Work out the finished part from the listing and answer in its coordinate system (mm). A direction names the side the tool comes from. Coordinates: 2 decimals unless noted, no trailing zeros. Order: outer loops, then holes, each group sorted by start corner. A loop starts at its lowest first (then second) coordinate and runs counter-clockwise, first axis right, second up. Notation, with made-up numbers: (3.25, -37.5) -> (32.25, -37.5) arc R16 ccw to (32.25, -19.5) -> close; hole circle Ø10 at (61.25, 43.25). An arc over 180 degrees is marked (long way). Write item = value, one per line. Start each with the question number.
Q1. The part is cut by section C-C, the plane y = -16. Determine the outline of the cut face in (x, z).
Q2. Which of the six approach directions +Z, -Z, +X, -X, +Y, -Y give full straight-line access (tool end or side, diameter ignored) to faces 1 (the flat face through (249, 24.789, 29)), 2 (the flat face through (247.33, 20.74, 34.51)), 3 (the cylindrical face through (243.607, 30.111, 40.975))?
Q3. The part is cut by section A-A, the plane y = 14.5. Determine the outline of the cut face in (x, z).
Q4. For a pull along X with two mould halves and no side action, classify faces 4 (the cylindrical face through (243.607, -11.164, 40.975)), 5 (the flat face through (244, -18.721, 40)), 6 (the flat face through (249.63, 11, 42)) as +X half, -X half, draft (parallel to the pull), parting line (faces both ways), or undercut.
Q5. Straight lines are drawn through the part: L1, parallel to Y at x = 242.5, z = 40; L2, parallel to Z at x = 248, y = 35; L3, parallel to X at y = -19, z = 19. For each, find the intervals that lie inside material, in ascending order. Write a range as from..to.
Q6. Flat-ended cylindrical pins translate along their axes: pin 1 (1.1 mm diameter, centred on x = 248, z = 27, fed in from +Y); pin 2 (12 mm diameter, centred on x = 257.5, z = 10, fed in from +Y); pin 3 (1 mm diameter, centred on y = -15, z = 28, fed in from +X); pin 4 (12 mm diameter, centred on x = 253.5, z = 13.5, fed in from -Y). Find the tip coordinate at first contact, or state that the pin passes through.
Q7. The part is cut by section D-D, the plane x = 260. Determine the outline of the cut face in (y, z).
Q8. The part is cut by section B-B, the plane x = 241. Determine the outline of the cut face in (y, z), plus the area to 3 significant figures.
```python
from build123d import *
from build123d.topology import SkipClean

# Parameters (mm, degrees)
SKETCH1_R           = 1.397
SKETCH1_R_2         = 4.0005
BOSS_EXTRUDE1_DEPTH = 3.175
SKETCH2_W           = 31.75
SKETCH2_H           = 57.15
BOSS_EXTRUDE2_DEPTH = 3.175
CUT_EXTRUDE2_DEPTH  = 3.175
CUT_EXTRUDE3_START  = 2.54
SKETCH4_R           = 23.6982
CUT_EXTRUDE3_DEPTH  = 2.54
SKETCH5_W           = 14.873793878
SKETCH5_H           = 32.130520557
CUT_EXTRUDE4_DEPTH  = 2.54
BOSS_EXTRUDE3_DEPTH = 2.54
SKETCH9_R           = 1.905
CUT_EXTRUDE6_DEPTH  = 6.35


with BuildPart() as part:
    # Sketch1 → Boss-Extrude1 (new body)
    # profile 1 of 2: a face of its own
    with BuildSketch(Plane(origin=(250.96748785, 0, 12.493901655), x_dir=(-0.04972137386865806, 0, 0.9987631275635946), z_dir=(-0.9987631275635946, -1.0338951916821772e-15, -0.04972137386865806))):
        with BuildLine():
            ThreePointArc((-0.642468938, 23.635575071), (-7.278200133, -18.075315821), (30.358231062, 1.090549523))
            ThreePointArc((30.358231062, 1.090549523), (25.825896406, 15.028780719), (13.962531062, 23.635575071))
            Line((13.962531062, 23.635575071), (13.962531062, 22.014532559))
            ThreePointArc((13.962531062, 22.014532559), (6.660031062, 2.792349523), (-0.642468938, 22.014532559))
            Line((-0.642468938, 22.014532559), (-0.642468938, 23.635575071))
        make_face()
        with Locations((2.106642694, -8.980550477)):
            Circle(SKETCH1_R, mode=Mode.SUBTRACT)
        with Locations((24.103687951, -8.980550477)):
            Circle(SKETCH1_R, mode=Mode.SUBTRACT)
        with Locations((-10.783625826, -1.538350477)):
            Circle(SKETCH1_R, mode=Mode.SUBTRACT)
        with Locations((-4.338491566, -5.259450477)):
            Circle(SKETCH1_R_2, mode=Mode.SUBTRACT)
        with Locations((17.658553691, -5.259450477)):
            Circle(SKETCH1_R_2, mode=Mode.SUBTRACT)
        with Locations((11.21341943, -1.538350477)):
            Circle(SKETCH1_R, mode=Mode.SUBTRACT)
    # profile 2 of 2: a face of its own
    with BuildSketch(Plane(origin=(250.96748785, 0, 12.493901655), x_dir=(-0.04972137386865806, 0, 0.9987631275635946), z_dir=(-0.9987631275635946, -1.0338951916821772e-15, -0.04972137386865806))):
        with BuildLine():
            Line((13.962531062, 22.014532559), (13.962531062, 23.635575071))
            ThreePointArc((13.962531062, 23.635575071), (6.660031062, 24.788749523), (-0.642468938, 23.635575071))
            Line((-0.642468938, 23.635575071), (-0.642468938, 22.014532559))
            ThreePointArc((-0.642468938, 22.014532559), (6.660031062, 2.792349523), (13.962531062, 22.014532559))
        make_face()
        with Locations((6.660031062, 13.790549523)):
            Circle(SKETCH1_R_2, mode=Mode.SUBTRACT)
        with Locations((0.214896802, 17.511649523)):
            Circle(SKETCH1_R, mode=Mode.SUBTRACT)
        with Locations((13.105165323, 10.069449523)):
            Circle(SKETCH1_R, mode=Mode.SUBTRACT)
    extrude(amount=BOSS_EXTRUDE1_DEPTH)

    # Sketch2 → Boss-Extrude2 (add)
    with BuildSketch(Plane(origin=(0, 0, 42.540622794), x_dir=(-1, 0, 0), z_dir=(0, 0, -1))):
        with Locations((-250.630940448, 9.853549523)):
            Rectangle(SKETCH2_W, SKETCH2_H)
    extrude(amount=BOSS_EXTRUDE2_DEPTH)

    # Sketch3 → Cut-Extrude2 (cut)
    with BuildSketch(Plane(origin=(0, 0, 39.365622794), x_dir=(-1, 0, 0), z_dir=(0, 0, -1))):
        Polygon((-249.629734326, 13.40907008), (-266.505940448, 22.553549523), (-266.505940448, -18.721450477), (-249.629734326, -18.721450477), align=None)
    extrude(amount=-CUT_EXTRUDE2_DEPTH, mode=Mode.SUBTRACT)

    # Sketch4 → Cut-Extrude3 (cut)
    with SkipClean():  # the faces are left unmerged after this step: merging them gives an invalid solid
        with BuildSketch(Plane(origin=(250.96748785, 0, 12.493901655), x_dir=(0.049721373868658096, 0, -0.9987631275635946), z_dir=(0.9987631275635946, 1.3357370765021432e-15, 0.049721373868658096)).offset(CUT_EXTRUDE3_START)):
            with Locations((-6.660031062, 1.090549523)):
                Circle(SKETCH4_R)
        extrude(amount=-CUT_EXTRUDE3_DEPTH, mode=Mode.SUBTRACT)

    # Sketch5 → Cut-Extrude4 (cut)
    with SkipClean():  # the faces are left unmerged after this step: merging them gives an invalid solid
        with BuildSketch(Plane.XY.offset(42.540622794)):
            with Locations((242.192837387, -2.656190199)):
                Rectangle(SKETCH5_W, SKETCH5_H)
        extrude(amount=CUT_EXTRUDE4_DEPTH, mode=Mode.SUBTRACT)

    # Sketch6 → Boss-Extrude3 (add)
    with BuildSketch(Plane(origin=(250.96748785, 0, 12.493901655), x_dir=(0.049721373868658096, 0, -0.9987631275635946), z_dir=(0.9987631275635946, 1.335737076502143e-15, 0.049721373868658096))):
        with BuildLine():
            ThreePointArc((-26.904999191, 13.40907008), (-18.272048961, 21.748858349), (-6.660031062, 24.788749523))
            Line((-6.660031062, 24.788749523), (-30.076072121, 24.788749523))
            Line((-30.076072121, 24.788749523), (-30.076072121, 13.40907008))
            Line((-30.076072121, 13.40907008), (-30.076072121, 4.736602785))
            ThreePointArc((-30.076072121, 4.736602785), (-28.91702666, 9.228782144), (-26.904999191, 13.40907008))
        make_face()
        with BuildLine():
            Line((-30.076072121, -2.55550374), (-30.076072121, -18.721450477))
            Line((-30.076072121, -18.721450477), (-19.663466733, -18.721450477))
            ThreePointArc((-19.663466733, -18.721450477), (-23.70122079, -15.377678552), (-26.904999191, -11.227971035))
            ThreePointArc((-26.904999191, -11.227971035), (-28.91702666, -7.047683098), (-30.076072121, -2.55550374))
        make_face()
    extrude(amount=-BOSS_EXTRUDE3_DEPTH)

    # Sketch9 → Cut-Extrude6 (cut)
    with BuildSketch(Plane.XY.offset(42.540622794)):
        with Locations((260.839665535, 29.538549523)):
            Circle(SKETCH9_R)
        with Locations((241.789665535, 29.538549523)):
            Circle(SKETCH9_R)
        with Locations((241.789665535, -11.736450477)):
            Circle(SKETCH9_R)
    extrude(amount=-CUT_EXTRUDE6_DEPTH, mode=Mode.SUBTRACT)


solid = part.part
```
Model answer:
q1.outline = (234.76, 39.37) -> (247.09, 39.37) -> (247.28, 35.42) -> (246.65, 35.38) -> (248.28, 2.59) -> (251.45, 2.75) -> (249.63, 39.37) -> (249.63, 42.54) -> (234.76, 42.54) -> close
q2.face_1 = -Z, +X, -X, +Y
q2.face_2 = -X, +Y
q2.face_3 = +Z, -Z
q3.outline = (234.76, 39.37) -> (247.09, 39.37) -> (247.13, 38.53) -> (246.49, 38.5) -> (247.27, 22.92) -> (250.44, 23.08) -> (249.63, 39.37) -> (251.64, 39.37) -> (251.64, 42.54) -> (234.76, 42.54) -> close; (247.66, 15.06) -> (248.44, -0.53) -> (251.61, -0.37) -> (250.83, 15.21) -> close
q4.face_4 = undercut
q4.face_5 = draft
q4.face_6 = +X half
q5.L1 = -18.72..-13.5, -9.97..27.77, 31.31..38.43
q5.L2 = 39.37..42.54
q5.L3 = 247.46..250.64
q6.pin_1 = 24.79
q6.pin_2 = through
q6.pin_3 = 250.22
q6.pin_4 = -22.6
q7.outline = (19.03, 39.37) -> (27.83, 39.37) -> (27.83, 42.54) -> (19.03, 42.54) -> close; (31.25, 39.37) -> (38.43, 39.37) -> (38.43, 42.54) -> (31.25, 42.54) -> close
q8.outline = (-18.72, 39.37) -> (-13.47, 39.37) -> (-13.47, 42.54) -> (-18.72, 42.54) -> close; (-10, 39.37) -> (27.8, 39.37) -> (27.8, 42.54) -> (-10, 42.54) -> close; (31.27, 39.37) -> (38.43, 39.37) -> (38.43, 42.54) -> (31.27, 42.54) -> close
q8.area = 159 mm2
